For this review, take the finished solid that the model builds, in its own axes (mm). A direction names the side the tool comes from. Coordinates: 2 decimals unless noted, no trailing zeros. Order: outer loops, then holes, each group sorted by start corner. A loop starts at its lowest first (then second) coordinate and runs counter-clockwise, first axis right, second up.
from build123d import *

# Parameters (mm, degrees)
CUT_EXTRUDE1_DEPTH  = 44.370496884
CIRPATTERN1_COUNT   = 25
SKETCH3_R           = 7.5
CUT_EXTRUDE2_DEPTH  = 43.84000856
CIRPATTERN2_COUNT   = 5
BOSS_EXTRUDE1_START = 1
SKETCH4_R           = 31
SKETCH4_R_2         = 25
BOSS_EXTRUDE1_DEPTH = 1
BOSS_EXTRUDE2_START = 5
SKETCH5_R           = 4.7
SKETCH5_R_2         = 2.7
BOSS_EXTRUDE2_DEPTH = 5


with BuildPart() as part:
    # Sketch1 → Revolve1 (revolve)
    with BuildSketch(Plane(origin=(0, 0, 0), x_dir=(0, 0, -1), z_dir=(1, 0, 0)), mode=Mode.PRIVATE) as revolve1_sk:
        Polygon((-4.5, 25), (-1.5, 25), (-1.5, 2.7), (1.5, 2.7), (1.5, 25), (4.5, 25), (4.5, 30), (-4.5, 30), align=None)
    revolve(revolve1_sk.sketch.rotate(Axis((0, 0, 3.054222254), (0, 0, -1)), 90), axis=Axis((0, 0, 3.054222254), (0, 0, -1)))

    # Sketch2 → Cut-Extrude1 (cut, through all)
    with BuildSketch(Plane(origin=(0, 0, -4.5), x_dir=(-1, 0, 0), z_dir=(0, 0, -1))):
        with BuildLine():
            ThreePointArc((0.450015258, 27.99638345), (-0.18373464, 27.999397165), (-0.817390411, 27.988066616))
            ThreePointArc((-0.817390411, 27.988066616), (-1.770903861, 29.232790202), (-3.222137334, 29.826461926))
            ThreePointArc((-3.222137334, 29.826461926), (-0.243371977, 29.999012818), (2.73780082, 29.874812914))
            ThreePointArc((2.73780082, 29.874812914), (1.353306055, 29.228633271), (0.450015258, 27.99638345))
        make_face()
    cut_extrude1 = extrude(amount=-CUT_EXTRUDE1_DEPTH, mode=Mode.SUBTRACT)

    # CirPattern1: Cut-Extrude1 ×25 about axis
    cirpattern1_axis = Axis((0, 0, 0), (0, 0, 1))
    for i in range(1, CIRPATTERN1_COUNT):
        add(cut_extrude1.rotate(cirpattern1_axis, i * 360 / CIRPATTERN1_COUNT), mode=Mode.SUBTRACT)

    # Sketch3 → Cut-Extrude2 (cut, through all)
    with BuildSketch(Plane(origin=(0, 0, -1.5), x_dir=(-1, 0, 0), z_dir=(0, 0, -1))):
        with Locations((0, 15.5)):
            Circle(SKETCH3_R)
    cut_extrude2 = extrude(amount=-CUT_EXTRUDE2_DEPTH, mode=Mode.SUBTRACT)

    # CirPattern2: Cut-Extrude2 ×5 about axis
    cirpattern2_axis = Axis((0, 0, 0), (0, 0, 1))
    for i in range(1, CIRPATTERN2_COUNT):
        add(cut_extrude2.rotate(cirpattern2_axis, i * 360 / CIRPATTERN2_COUNT), mode=Mode.SUBTRACT)

    # Sketch4 → Boss-Extrude1 (add)
    with BuildSketch(Plane(origin=(0, 0, -4.5), x_dir=(-1, 0, 0), z_dir=(0, 0, -1)).offset(BOSS_EXTRUDE1_START)):
        Circle(SKETCH4_R)
        with Locations(Location((0, 0, 0), (0, 0, 180))):
            Circle(SKETCH4_R_2, mode=Mode.SUBTRACT)
    boss_extrude1 = extrude(amount=-BOSS_EXTRUDE1_DEPTH)

    # Sketch5 → Boss-Extrude2 (add)
    with BuildSketch(Plane(origin=(0, 0, -1.5), x_dir=(-1, 0, 0), z_dir=(0, 0, -1)).offset(BOSS_EXTRUDE2_START)):
        with Locations(Location((0, 0, 0), (0, 0, 180))):
            Circle(SKETCH5_R)
        with Locations(Location((0, 0, 0), (0, 0, 180))):
            Circle(SKETCH5_R_2, mode=Mode.SUBTRACT)
    boss_extrude2 = extrude(amount=-BOSS_EXTRUDE2_DEPTH)

    # Mirror2: Boss-Extrude2 across plane
    add(boss_extrude2.mirror(Plane.XY))

    # Mirror3: Boss-Extrude1 across plane
    add(boss_extrude1.mirror(Plane.XY))


solid = part.part
1. Take a section at A-A, the plane z = 3.5. Give the number of separate pieces and of enclosed holes in the cut face, plus the area to 3 significant figures.
Answer below:
separate pieces: 2
enclosed holes: 2
area: 768 mm2
2. Machinability: for faces 1 (the face through (-12.387, -26.522, -0.063)), 2 (the face through (27.39, 10.34, -0.06)), 3 (the face through (-21.02, 20.38, -0.06)), 4 (the face through (-23.73, 17.14, -0.06)), 5 (the face through (0, 5, -1.5)), which of the approach directions +Z, -Z, +X, -X, +Y, -Y give a long, thin tool a straight path to every point of the face, cutting with its end or side? Answer none if there is none.
Answer below:
face 1: -Y
face 2: +X
face 3: +Y
face 4: -X
face 5: -Z
3. Take a section at B-B, the plane y = -24. Give the boundary of the cut face in (x, z), plus the area to 3 significant figures.
Answer below:
outline: (-19.62, -5.5) - (-7, -5.5) - (-7, -1.5) - (7, -1.5) - (7, -5.5) - (19.62, -5.5) - (19.62, -4.5) - (15.87, -4.5) - (15.87, 4.5) - (19.62, 4.5) - (19.62, 5.5) - (7, 5.5) - (7, 1.5) - (-7, 1.5) - (-7, 5.5) - (-19.62, 5.5) - (-19.62, 4.5) - (-16.17, 4.5) - (-16.17, -4.5) - (-19.62, -4.5) - close
area: 255 mm2
4. Clearance check with flat-ended pins moving along their axes: pin 1 Ø1 at (x, z) = (-2, 2.5) entering from -Y; pin 2 Ø5 at (x, y) = (5.5, 11.5) entering from -Z; pin 3 Ø5 at (y, z) = (19, -4) entering from -X. State where each tip first meets the part, or that it passes through.
Answer below:
pin 1: stops at y = -29.79
pin 2: stops at z = -1.5
pin 3: stops at x = -26.21
5. To check wall thickness, follow L1, parallel to Y at x = -1.5, z = -3 (3 decimals); L2, parallel to Y at x = 0, z = 4.8; L3, parallel to Z at x = -11, y = 28.5. State the ranges of each line that lie inside material, in increasing order.
Answer below:
L1: y = -29.786 to -24.955, -4.454 to -2.245, 2.245 to 4.454, 24.955 to 29.342
L2: y = -31 to -25, -4.7 to -2.7, 2.7 to 4.7, 25 to 31
L3: z = -5.5 to -4.5, 4.5 to 5.5
6. The part is to be moulded in two halves that separate along Y. For faces 6 (the face through (-23.631, -17.274, -0.063)), 7 (the face through (-3.53, 29.79, 0.06)), 8 (the face through (23.956, 16.826, -0.063)), 9 (the face through (28.33, 7.36, -0.06)), say which applies: +Y half, -Y half, draft (parallel to the pull), parting line (faces both ways), or undercut.
Answer below:
face 6: -Y half
face 7: +Y half
face 8: undercut
face 9: undercut
